```python
from build123d import *

# Parameters (mm, degrees)
PAD002_DEPTH = 3
FILLET003_R  = 1


with BuildPart() as revolution001:
    # Sketch005 → Revolution001 (revolve)
    with BuildSketch(Plane.XZ):
        Polygon((0, 0), (7.5, 0), (7.5, 1), (3, 1), (3, 135.736657), (0, 135.736657), align=None)
    revolve(axis=Axis((0, 0, 0), (0, 0, 1)))


with BuildPart() as pad002:
    # Pad002 base: copy of Revolution001
    add(revolution001.part)

    # Sketch006 → Pad002 (new body)
    with BuildSketch(Plane(origin=(0, 0, 1), x_dir=(-1, 0, 0), z_dir=(0, 0, 1))):
        Polygon((-5, 1), (-5, -1), (-1, -1), (-1, -5), (1, -5), (1, -1), (5, -1), (5, 1), (1, 1), (1, 5), (-1, 5), (-1, 1), align=None)
    extrude(amount=PAD002_DEPTH)


with BuildPart() as fillet003:
    # Fusion001 base: copy of Revolution001
    add(revolution001.part)

    # Fusion001: union Pad002
    add(pad002.part)

    # Fillet003
    fillet003_edges = [fillet003.edges().sort_by_distance(p)[0] for p in [
        (0, 5, 4),
        (-5, 0, 4),
        (0, -5, 4),
        (5, 0, 4),
    ]]
    fillet(fillet003_edges, radius=FILLET003_R)


solid = fillet003.part
```
The listing builds one solid part. Answer for the finished solid, in the listing's coordinates (mm). A direction names the side the tool comes from. Give positions to 0.01 mm unless a question says otherwise; leave off trailing zeros. Write each loop counter-clockwise with the first axis right and the second up, starting at its lowest first coordinate (ties: lowest second). Pieces come first, ordered by that corner, then holes. Notation, with made-up numbers: (61.5, 68) - (108.5, 68) arc R21 cw to (108.5, 105) - close; hole circle Ø10 at (42.5, -18.5). An arc over 180 degrees is marked (long way). Use one line per item in the form item = value. Start each with the question number.
1) Consider line 1 along Z through (x, y) = (2.75, 6.5); line 2 along Y through (x, z) = (0.25, 96); line 3 along X through (y, z) = (-1, 78.5). Determine where each line is inside the solid, lowest interval first. Write a range as from..to.
2) Flat-ended cylindrical pins translate along their axes: pin 1 Ø3 at (y, z) = (0, 62.5) entering from -X; pin 2 Ø8 at (y, z) = (0.5, 36) entering from +X; pin 3 Ø1.7 at (x, z) = (-3.5, 2) entering from -Y. Find the tip coordinate at first contact, or state that the pin passes through.
3) A tool of negligible diameter and unlimited length cuts with its end or side. For faces 1 (the face through (4, 1, 2)), 2 (the face through (-1, 4, 2)), 3 (the face through (-1, -4, 2)), from which of +Z, -Z, +X, -X, +Y, -Y can it reach the whole face along a straight path? Write none if from no direction.
4) Find section A-A on z = 12.5. Determine the outline of the cut face in (x, y), plus the area to 3 significant figures.
Geometry results:
q1.line_1 = 0..1
q1.line_2 = -2.99..2.99
q1.line_3 = -2.83..2.83
q2.pin_1 = -3
q2.pin_2 = 3
q2.pin_3 = -1.41
q3.face_1 = +Z, +X, +Y
q3.face_2 = +Z, -X, +Y
q3.face_3 = +Z, -X, -Y
q4.outline = circle Ø6 at (0, 0)
q4.area = 28.3 mm2
